from build123d import *

# Parameters (mm, degrees)
CROQUIS1_W                 = 3.5
CROQUIS1_H                 = 9
CROQUIS1_H_2               = 4
CROQUIS1_W_2               = 5.00348191
CROQUIS1_H_3               = 3.000000003
SALIENTE_EXTRUIR1_DEPTH    = 3
S_LIDO_MOVER_COPIAR1_ANGLE = 90


with BuildPart() as part:
    # Croquis1 → Saliente-Extruir1 (new body)
    with BuildSketch(Plane.XY):
        Polygon((-323.234450912, 58307.505235193), (-323.234450912, 58304.505235193), (-321.699124199, 58304.505235193), (-321.699124199, 58301.505235193), (-322.699124199, 58301.505235193), (-322.699124199, 58299.505235193), (-321.699124199, 58299.505235193), (-321.699124199, 58295.505235193), (-318.699124199, 58295.505235193), (-318.699124199, 58299.505235193), (-317.699124199, 58299.505235193), (-317.699124199, 58301.505235193), (-318.699124199, 58301.505235193), (-318.699124199, 58304.505235193), (-316.699124199, 58304.505235193), (-316.699124199, 58307.505235193), (-310.234450912, 58307.505235193), (-310.234450912, 58259.505235194), (-310.699124199, 58259.505235194), (-310.699124199, 58256.505235193), (-315.699124199, 58256.505235193), (-315.699124199, 58259.505235193), (-318.699124199, 58259.505235193), (-318.699124199, 58262.505235193), (-317.699124199, 58262.505235193), (-317.699124199, 58264.505235193), (-318.699124199, 58264.505235193), (-318.699124199, 58268.505235193), (-321.699124199, 58268.505235193), (-321.699124199, 58264.505235193), (-322.699124199, 58264.505235193), (-322.699124199, 58262.505235193), (-321.699124199, 58262.505235193), (-321.699124199, 58259.505235193), (-323.699124199, 58259.505235193), (-323.699124199, 58256.505235193), (-326.699124199, 58256.505235193), (-326.699124199, 58259.505235193), (-327.699124199, 58259.505235193), (-327.699124199, 58256.505235193), (-330.699124199, 58256.505235193), (-330.699124199, 58259.505235194), (-331.234450912, 58259.505235194), (-331.234450912, 58304.505235193), (-330.234450912, 58304.505235193), (-330.234450912, 58307.505235193), align=None)
        with Locations((-324.949124199, 58286.005235193)):
            Rectangle(CROQUIS1_W, CROQUIS1_H, mode=Mode.SUBTRACT)
        with Locations((-314.949124199, 58286.005235193)):
            Rectangle(CROQUIS1_W, CROQUIS1_H_2, mode=Mode.SUBTRACT)
        with Locations((-319.697383244, 58278.005235192)):
            Rectangle(CROQUIS1_W_2, CROQUIS1_H_3, mode=Mode.SUBTRACT)
    extrude(amount=SALIENTE_EXTRUIR1_DEPTH)


with BuildPart() as part_1:
    # Sólido-Mover/Copiar1: moved
    add(part.part.rotate(Axis((0, 58282.005235193, 1.5), (1, 0, 0)), S_LIDO_MOVER_COPIAR1_ANGLE))


solid = part_1.part
Geometry check sheet. Reference: the model listing, model coordinates, mm. A direction names the side the tool comes from. Give positions to 0.01 mm unless a question says otherwise; leave off trailing zeros. Loops run counter-clockwise (first coordinate to the right, second up) from the corner with the lowest first, then second, coordinate; pieces in that order, holes last. Notation, with made-up numbers: M 51.25,54.5 L 73.25,54.5 A24 cw 73.25,83.5 Z; hole C 82.5,55.25 d9. An arc over 180 degrees is marked long. Answer as a JSON object with one key per item and string values. Group by question number.
Item 1: Material ranges on L1, parallel to Z at x = -322.25, y = 58282.65; L2, parallel to X at y = 58281.9, z = 5.5; L3, parallel to Z at x = -322, y = 58281.55, recorded low to high.
Item 2: Mould release check, pull along X, two halves, no side actions. Record for faces 5 (the flat face through (-310.234, 58282, 3)), 6 (the flat face through (-315, 58282, 3.5)), 7 (the flat face through (-321, 58280.505, 2)): pulls with the +X half, pulls with the -X half, needs draft (parallel to the pull), parting line crosses it, or undercut.
Item 3: Sectioned sample at B-B on z = -2.5. Record the boundary of the cut face in (x, y).
Item 4: Sectioned sample at A-A on x = -315. Record the boundary of the cut face in (y, z).
Item 5: Sectioned sample at C-C on y = 58281.7. Give the number of separate pieces and of enclosed holes in the cut face, plus the area to 3 significant figures.
Item 6: Access from +Z, -Z, +X, -X, +Y, -Y to the whole of each face (thin tool, end or side, straight path). Record for faces 1 (the flat face through (-321.699, 58282, 23)), 2 (the flat face through (-327, 58282, -21)), 3 (the flat face through (-331, 58282, 24)), 4 (the flat face through (-325, 58282, 1)).
Item 7: Gauge pin test, flat ends, axial feed: pin 1 (0.5 mm diameter, centred on x = -327, y = 58281.5, fed in from -Z); pin 2 (1.5 mm diameter, centred on x = -319.5, y = 58282.5, fed in from +Z). Record the tip position at first contact, or that the pin passes through.
Findings below:
{
 "1": {"L1": "-21 to -18, -16 to 19, 21 to 24", "L2": "-331.23 to -326.7, -323.2 to -316.7, -313.2 to -310.23", "L3": "-21 to -18, -16 to -4, -1 to 19, 21 to 24"},
 "2": {"face 5": "pulls with the +X half", "face 6": "undercut", "face 7": "needs draft"},
 "3": {"outline": "M -331.23,58280.51 L -322.2,58280.51 L -322.2,58283.51 L -331.23,58283.51 Z; M -317.2,58280.51 L -310.23,58280.51 L -310.23,58283.51 L -317.2,58283.51 Z"},
 "4": {"outline": "M 58280.51,-24 L 58283.51,-24 L 58283.51,3.5 L 58280.51,3.5 Z; M 58280.51,7.5 L 58283.51,7.5 L 58283.51,27 L 58280.51,27 Z"},
 "5": {"separate pieces": "1", "enclosed holes": "3", "area": "896 mm2"},
 "6": {"face 1": "+Z, +Y, -Y", "face 2": "-Z, +Y, -Y", "face 3": "+Z, -X, +Y, -Y", "face 4": "+Y, -Y"},
 "7": {"pin 1": "z = -21", "pin 2": "z = 15"}
}
